Source: CAD feature listing. Evaluate the final solid. Frame: model axes, mm. A direction names the side the tool comes from. Give positions to 0.01 mm unless a question says otherwise; leave off trailing zeros. Loops run counter-clockwise (first coordinate to the right, second up) from the corner with the lowest first, then second, coordinate; pieces in that order, holes last. Notation, with made-up numbers: (88.5, 46.25) -> (132.5, 46.25) arc R36 cw to (132.5, 84.25) -> close; hole circle Ø4 at (-14, 9). An arc over 180 degrees is marked (long way). Return JSON: item names as keys, results as strings. Group by question number.
(1) Draft query along Y for faces 1 (the face through (85, 20.107, 5)), 2 (the face through (-9.031, -8.642, 4.93)), 3 (the face through (5.887, 22.181, 4.93)), 4 (the face through (33, 18.1, 5.1)). Return one class per face: released by +Y, released by -Y, zero draft, split by the parting line, or undercut.
(2) Cut plane C-C on x = 170. Return loops of the section in (y, z) (3 decimals).
(3) Cut plane B-B on z = 2.25. Give the number of separate pieces and of enclosed holes in the cut face, then the cut area to 3 significant figures.
(4) Pin query (flat end, axial travel): pin 1 (5 mm diameter, centred on x = 27, z = 4.5, fed in from -Y); pin 2 (10.5 mm diameter, centred on x = 0, y = 0, fed in from -Z); pin 3 (1 mm diameter, centred on y = -7.5, z = 4.5, fed in from +X); pin 4 (1 mm diameter, centred on y = 3, z = 2, fed in from +X). Return the tip coordinate at first contact, or that it passes through.
(5) Access query for faces 5 (the face through (173.46, 14.22, 4.93)), 6 (the face through (12.36, -5.32, 4.93)), 7 (the face through (145, 16.107, 5)). Directions: +Z, -Z, +X, -X, +Y, -Y. A direction counts if a zero-diameter tool reaches every point of the face in a straight line with its end or side. Return the directions, or none.
(6) Cut plane A-A on x = 25. Return loops of the section in (y, z).
(7) Ray query, line 1 (Y direction, x = 104, z = 6); line 2 (X direction, y = 1, z = 6); line 3 (Y direction, x = 0, z = 3). Return the intervals inside material, ascending. Write a range as from..to.
```python
from build123d import *

# Parameters (mm, degrees)
SKETCH_R               = 6.5
SKETCH_R_2             = 2.425
PAD_DEPTH              = 10
POCKET_DEPTH           = 15
LINEARPATTERN_COUNT    = 4
LINEARPATTERN_PITCH    = 20
LINEARPATTERN001_COUNT = 4
LINEARPATTERN001_PITCH = 20


with BuildPart() as part:
    # Sketch → Pad (new body)
    with BuildSketch(Plane.XY):
        with BuildLine():
            ThreePointArc((-8.838835, 8.838835), (-8.838835, -8.838835), (8.838835, -8.838835))
            Line((15.784271, -1.893398), (8.838835, -8.838835))
            Line((15.784271, -1.893398), (154.215729, -1.893398))
            Line((154.215729, -1.893398), (161.161165, -8.838835))
            ThreePointArc((161.161165, -8.838835), (178.838835, -8.838835), (178.838835, 8.838835))
            Line((168.232233, 19.445436), (178.838835, 8.838835))
            ThreePointArc((168.232233, 19.445436), (164.176941, 22.155096), (159.393398, 23.106602))
            Line((10.606602, 23.106602), (159.393398, 23.106602))
            ThreePointArc((10.606602, 23.106602), (5.823059, 22.155096), (1.767767, 19.445436))
            Line((-8.838835, 8.838835), (1.767767, 19.445436))
        make_face()
        Circle(SKETCH_R, mode=Mode.SUBTRACT)
        with Locations((170, 0)):
            Circle(SKETCH_R_2, mode=Mode.SUBTRACT)
    extrude(amount=PAD_DEPTH)

    # Sketch001 (on Face14 of Pad) → Pocket (cut)
    with BuildSketch(Plane.XY.offset(10)):
        with BuildLine():
            ThreePointArc((79, 20.106602), (77, 18.106602), (79, 16.106602))
            Line((79, 16.106602), (91, 16.106602))
            ThreePointArc((91, 16.106602), (93, 18.106602), (91, 20.106602))
            Line((91, 20.106602), (79, 20.106602))
        make_face()
    pocket = extrude(amount=-POCKET_DEPTH, mode=Mode.SUBTRACT)

    # LinearPattern: Pocket ×4
    with Locations(*[(i * LINEARPATTERN_PITCH, 0, 0) for i in range(1, LINEARPATTERN_COUNT)]):
        add(pocket, mode=Mode.SUBTRACT)

    # LinearPattern001: Pocket ×4
    with Locations(*[(-i * LINEARPATTERN001_PITCH, 0, 0) for i in range(1, LINEARPATTERN001_COUNT)]):
        add(pocket, mode=Mode.SUBTRACT)


solid = part.part
```
Answers:
{
 "1": {"face 1": "undercut", "face 2": "split by the parting line", "face 3": "released by +Y", "face 4": "undercut"},
 "2": {"outline": "(-12.5, 0) -> (-2.425, 0) -> (-2.425, 10) -> (-12.5, 10) -> close; (2.425, 0) -> (17.678, 0) -> (17.678, 10) -> (2.425, 10) -> close"},
 "3": {"separate pieces": "1", "enclosed holes": "9", "area": "4,380 mm²"},
 "4": {"pin 1": "y = -1.89", "pin 2": "through", "pin 3": "x = 180.36", "pin 4": "x = 182.25"},
 "5": {"face 5": "+Z, -Z, +X, +Y", "face 6": "+Z, -Z, -Y", "face 7": "+Z, -Z"},
 "6": {"outline": "(-1.89, 0) -> (16.11, 0) -> (16.11, 10) -> (-1.89, 10) -> close; (20.11, 0) -> (23.11, 0) -> (23.11, 10) -> (20.11, 10) -> close"},
 "7": {"line 1": "-1.89..16.11, 20.11..23.11", "line 2": "-12.46..-6.42, 6.42..167.79, 172.21..182.46", "line 3": "-12.5..-6.5, 6.5..17.68"}
}
